Source: three-view drawing plus pictorial views. Frame: mm from the lowest corner of the part. A direction names the side the tool comes from. Give positions to 0.01 mm unless a question says otherwise; leave off trailing zeros. Order: outer loops, then holes, each group sorted by start corner. A loop starts at its lowest first (then second) coordinate and runs counter-clockwise, first axis right, second up.
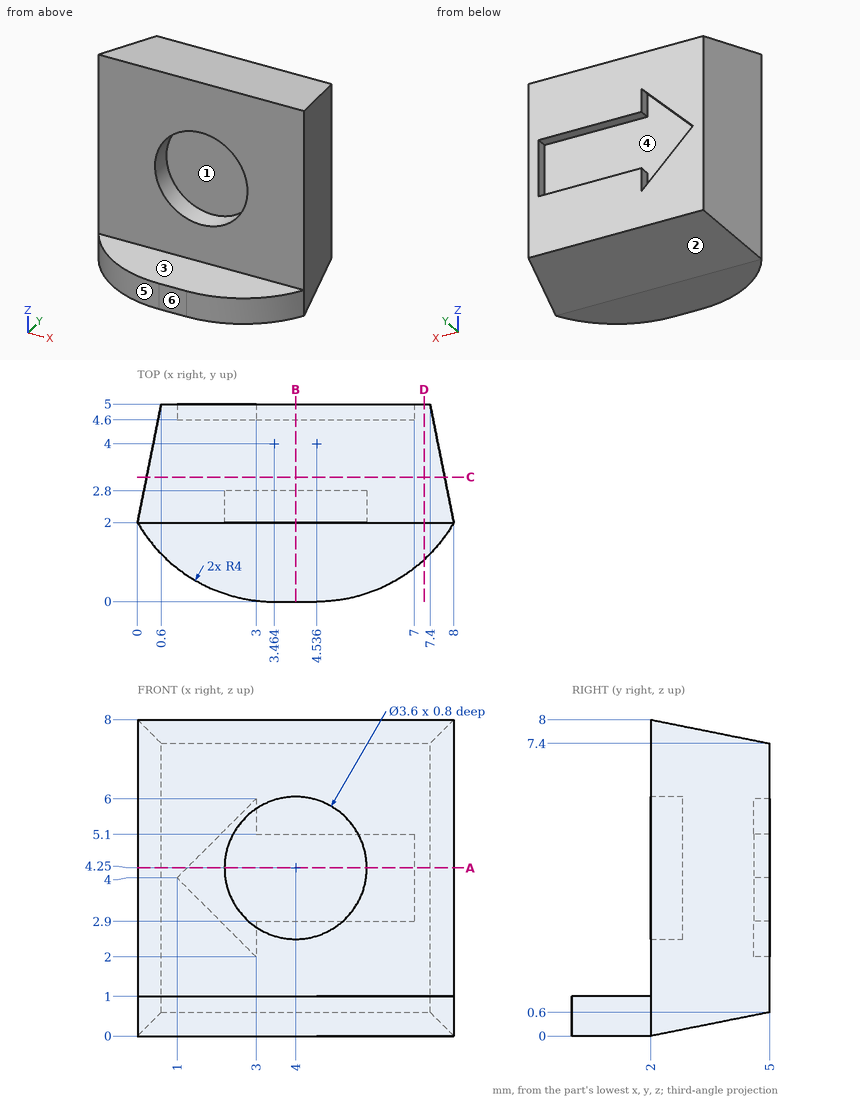
1) Ray query, L1, parallel to Y at x = 1.75, z = 3.5; L2, parallel to X at y = 2.35, z = 4.25; L3, parallel to Y at x = 1.75, z = 1.25. Return the intervals inside material, ascending.
Checks:
L1: y = 2 to 4.6
L2: x = 0.07 to 2.2, 5.8 to 7.93
L3: y = 2 to 5
2) Reachability of the marked faces 1, 2 and 3 from +Z, -Z, +X, -X, +Y, -Y: full face, straight path, thin tool, end or side. Return the list, or none.
Checks:
face 1: -Y
face 2: -Z, +X, -X, +Y
face 3: +Z, +X, -X, -Y
3) Section query D-D on x = 7.25. Output: boundary loops of the cut face in (y, z), and give its area (3 significant figures).
Checks:
outline: (1.06, 0) - (2, 0) - (5, 0.6) - (5, 7.4) - (2, 8) - (2, 1) - (1.06, 1) - close
area: 23.1 mm2
4) Pull-direction query (X, two-part tool) for the marked faces 4, 5 and 6; classes: +X half, -X half, draft (parallel to the pull), parting line (faces both ways), or undercut.
Checks:
face 4: undercut
face 5: -X half
face 6: draft
5) Section query A-A on z = 4.25. Output: boundary loops of the cut face in (x, y).
Checks:
outline: (0, 2) - (2.2, 2) - (2.2, 2.8) - (5.8, 2.8) - (5.8, 2) - (8, 2) - (7.4, 5) - (7, 5) - (7, 4.6) - (1.25, 4.6) - (1.25, 5) - (0.6, 5) - close
6) Section query B-B on x = 4. Output: boundary loops of the cut face in (y, z), and give its area (3 significant figures).
Checks:
outline: (0, 0) - (2, 0) - (5, 0.6) - (5, 2.9) - (4.6, 2.9) - (4.6, 5.1) - (5, 5.1) - (5, 7.4) - (2, 8) - (2, 6.05) - (2.8, 6.05) - (2.8, 2.45) - (2, 2.45) - (2, 1) - (0, 1) - close
area: 20.4 mm2
7) Section query C-C on y = 3.15. Output: boundary loops of the cut face in (x, z).
Checks:
outline: (0.23, 0.23) - (7.77, 0.23) - (7.77, 7.77) - (0.23, 7.77) - close
8) First-contact query: pin 1 Ø1 at (x, z) = (6.5, 5) entering from -Y; pin 2 Ø0.6 at (x, y) = (4.5, 1.5) entering from +Z; pin 3 Ø1.8 at (x, z) = (4, 3.5) entering from -Y. Flat tips, straight axial feed; report the tip coordinate or a pass-through.
Checks:
pin 1: stops at y = 2
pin 2: stops at z = 1
pin 3: stops at y = 2.8
